Study the drawing (mm; zero at the part's minimum x, y, z) and answer. Coordinates: 2 decimals unless noted, no trailing zeros. Order: outer loops, then holes, each group sorted by start corner. A loop starts at its lowest first (then second) coordinate and runs counter-clockwise, first axis right, second up. Notation, with made-up numbers: (16.5, -18) -> (51.5, -18) arc R20 ccw to (51.5, 11) -> close; hole circle Ø11 at (2.5, -38). An arc over 180 degrees is marked (long way). Write each question's results on one line, items separated by ' | '. Start each with the question number.
(1) The part is cut by section C-C, the plane y = 3.75. Give the vertices of the cut face in (x, z), then the cut area to 3 significant figures.
(2) The part is cut by section D-D, the plane y = 5. Give the vertices of the cut face in (x, z).
(3) Determine the mould class of the marked faces 1, 2, 3 and 4 for opening direction X: +X half, -X half, draft (parallel to the pull), parting line (faces both ways), or undercut.
(4) Given pin 1 (1 mm diameter, centred on x = 8, y = 6, fed in from -Z); pin 2 (1 mm diameter, centred on y = 4.5, z = 10, fed in from +X); pin 3 (5.5 mm diameter, centred on x = 6, z = 6, fed in from -Y); pin 4 (4 mm diameter, centred on y = 3.5, z = 2, fed in from +X), each flat-ended and moving along its own axis, determine where each tip first touches the part or whether it passes through.
(5) Straight lines are drawn through the part: L1, parallel to X at y = 0.55, z = 6; L2, parallel to Z at x = 5, y = 3.75. For each, find the intervals that lie inside material, in ascending order.
(6) The part is cut by section B-B, the plane z = 6. Give the vertices of the cut face in (x, y), then the cut area to 3 significant figures.
(7) The part is cut by section A-A, the plane x = 6. Give the vertices of the cut face in (y, z), then the cut area to 3 significant figures.
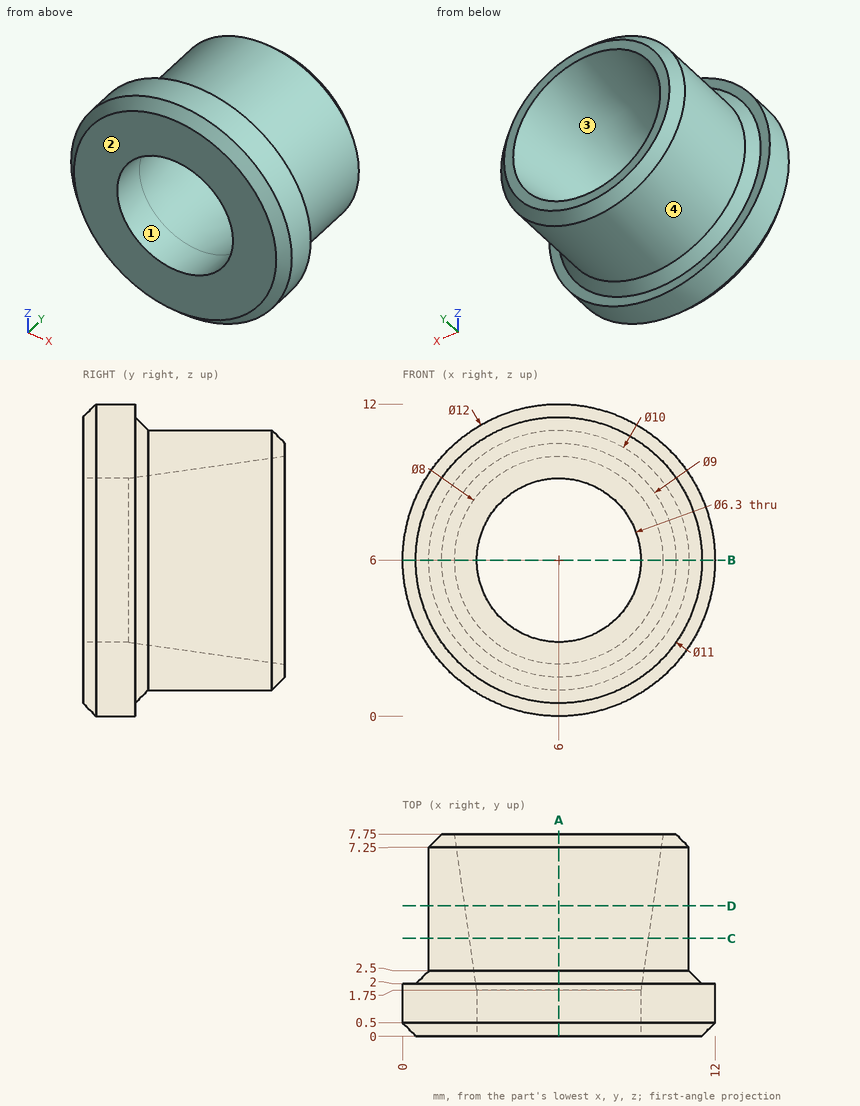
Established:
1) outline: circle Ø10 at (6, 6); hole circle Ø6.87 at (6, 6) | area: 41.5 mm^2
2) outline: circle Ø10 at (6, 6); hole circle Ø7.22 at (6, 6)
3) face 1: undercut | face 2: draft | face 3: undercut | face 4: parting line
4) pin 1: stops at z = 1.23 | pin 2: stops at x = 9.57 | pin 3: passes through | pin 4: stops at x = 11.37
5) L1: x = 0 to 2.85, 9.15 to 12 | L2: z = 1.1 to 2.72, 9.28 to 10.9
6) outline: (0, 0.5) -> (0.5, 0) -> (2.85, 0) -> (2.85, 1.75) -> (2, 7.75) -> (1.5, 7.75) -> (1, 7.25) -> (1, 2.5) -> (0.5, 2) -> (0, 2) -> close; (9.15, 0) -> (11.5, 0) -> (12, 0.5) -> (12, 2) -> (11.5, 2) -> (11, 2.5) -> (11, 7.25) -> (10.5, 7.75) -> (10, 7.75) -> (9.15, 1.75) -> close | area: 27.3 mm^2
7) outline: (0, 0.5) -> (0.5, 0) -> (2, 0) -> (2, 0.5) -> (2.5, 1) -> (7.25, 1) -> (7.75, 1.5) -> (7.75, 2) -> (1.75, 2.85) -> (0, 2.85) -> close; (0, 9.15) -> (1.75, 9.15) -> (7.75, 10) -> (7.75, 10.5) -> (7.25, 11) -> (2.5, 11) -> (2, 11.5) -> (2, 12) -> (0.5, 12) -> (0, 11.5) -> close | area: 27.3 mm^2
